Check sheet for the modelled part. Datum: model origin and axes. Units: mm. Give positions to 0.01 mm unless a question says otherwise; leave off trailing zeros. Loops run counter-clockwise (first coordinate to the right, second up) from the corner with the lowest first, then second, coordinate; pieces in that order, holes last. Notation, with made-up numbers: (14.5, -36) - (26.5, -36) arc R22 cw to (26.5, -30) - close; hole circle Ø8 at (58, -35). An arc over 180 degrees is marked (long way). Answer in a Markdown table with one row per item. Add a question column.
(1) Draft check along Z on faces 1 (the face through (-1.947, 0.119, -2.539)), 2 (the face through (2.839, 0.119, -2.817)), 3 (the face through (3.5, 0, 0)). Enter one of: released by +Z, released by -Z, zero draft, split by the parting line, or undercut.
(2) Thickness scan on L1, parallel to X at y = 5, z = 0; L2, parallel to Z at x = -1.5, y = -6.75. Record the ranges inside material, lowest first.
(3) Sectioned sample at A-A on z = 0. Enter the section's corners in (x, y).
(4) Sectioned sample at C-C on y = 2.5. Enter the section's corners in (x, z), then the cut area to 3 significant figures.
(5) Sectioned sample at B-B on x = 0. Enter the section's corners in (y, z).
Solid Edge part; units mm, degrees
sketch "Sketch1" plane through (0, 0, 0) normal (0, -1, 0) x (1, 0, 0)
  circle A0 centre (0, 0) radius 4
extrude "Protrusion1" add sketch "Sketch1" along normal mid plane 17
sketch "Sketch2" plane through (0, 8.5, 0) normal (0, 1, 0) x (0, 0, -1)
  line L0 (3.5, -3.5) -> (-3.5, -3.5)
  line L1 (-3.5, -3.5) -> (-3.5, 3.5)
  line L2 (-3.5, 3.5) -> (3.5, 3.5)
  line L3 (3.5, 3.5) -> (3.5, -3.5)
  line L4 (5, 5) -> (-5, 5)
  line L5 (-5, 5) -> (-5, -5)
  line L6 (-5, -5) -> (5, -5)
  line L7 (5, -5) -> (5, 5)
  dimension "D1" = 3.5
  dimension "D2" = 5
extrude "Cutout1" cut sketch "Sketch2" against normal through all
hole "Agujero_1" at (0, 8.5, 0) direction (0, -1, 0) diameter 6.4 end up to next
properties part number "1976-1500-008" material "Aluminio, 7075-T6"
Reply:
| question | item | result |
|---|---|---|
| 1 | face 1 | undercut |
| 1 | face 2 | released by -Z |
| 1 | face 3 | zero draft |
| 2 | L1 | -3.5 to -3.2, 3.2 to 3.5 |
| 2 | L2 | -3.5 to -2.83, 2.83 to 3.5 |
| 3 | outline | (-3.5, -8.5) - (-3.2, -8.5) - (-3.2, 8.5) - (-3.5, 8.5) - close; (3.2, -8.5) - (3.5, -8.5) - (3.5, 8.5) - (3.2, 8.5) - close |
| 4 | outline | (-3.5, -1.94) arc R4 ccw to (-1.94, -3.5) - (1.94, -3.5) arc R4 ccw to (3.5, -1.94) - (3.5, 1.94) arc R4 ccw to (1.94, 3.5) - (-1.94, 3.5) arc R4 ccw to (-3.5, 1.94) - close; hole circle Ø6.4 at (0, 0) |
| 4 | area | 12.9 mm^2 |
| 5 | outline | (-8.5, -3.5) - (8.5, -3.5) - (8.5, -3.2) - (-8.5, -3.2) - close; (-8.5, 3.2) - (8.5, 3.2) - (8.5, 3.5) - (-8.5, 3.5) - close |
